The listing builds one solid part. Answer for the finished solid, in the listing's coordinates (mm). A direction names the side the tool comes from. Coordinates: 2 decimals unless noted, no trailing zeros. Loops run counter-clockwise (first coordinate to the right, second up) from the corner with the lowest first, then second, coordinate; pieces in that order, holes last. Notation, with made-up numbers: (43.5, 12) -> (81.5, 12) arc R10 ccw to (81.5, 30) -> close; hole circle Ø4 at (7.25, 39.25). An arc over 180 degrees is marked (long way). Answer in a Markdown table with one row per item.
```python
from build123d import *

# Parameters (mm, degrees)
AXIAL_PROFILE_MM_W     = 5
AXIAL_PROFILE_MM_H     = 34.4
AXIAL_HOLES_DEPTH      = 176.574514096
AXIAL_HOLES_DEPTH_BACK = 176.574514096
SKETCH2_R              = 1.65
CUT_EXTRUDE2_START     = 165.2
SKETCH3_R              = 1.65
CUT_EXTRUDE2_DEPTH     = 3.5


with BuildPart() as part:
    # Axial profile (mm) → Full revolution (revolve)
    with BuildSketch(Plane.XY, mode=Mode.PRIVATE) as full_revolution_sk:
        with Locations((166.2, 17.2)):
            Rectangle(AXIAL_PROFILE_MM_W, AXIAL_PROFILE_MM_H)
    revolve(full_revolution_sk.sketch.rotate(Axis((-110, 0, 0), (1, 0, 0)), 90), axis=Axis((-110, 0, 0), (1, 0, 0)))

    # Sketch2 → Axial holes (cut, two sides: drawn at the far end of the back side and taken through both)
    with BuildSketch(Plane(origin=(0, 0, 0), x_dir=(0, 0, -1), z_dir=(1, 0, 0)).offset(-AXIAL_HOLES_DEPTH_BACK)):
        with Locations((-29.4, 0)):
            Circle(SKETCH2_R)
        with Locations((14.7, -25.461146871)):
            Circle(SKETCH2_R)
        with Locations((14.7, 25.461146871)):
            Circle(SKETCH2_R)
    extrude(amount=AXIAL_HOLES_DEPTH + AXIAL_HOLES_DEPTH_BACK, mode=Mode.SUBTRACT)

    # Sketch3 → Cut-Extrude2 (cut)
    with BuildSketch(Plane(origin=(0, 0, 0), x_dir=(0, 0, -1), z_dir=(1, 0, 0)).offset(CUT_EXTRUDE2_START)):
        with Locations((29.4, 0)):
            Circle(SKETCH3_R)
        with Locations((-14.7, 25.461146871)):
            Circle(SKETCH3_R)
        with Locations((-14.7, -25.461146871)):
            Circle(SKETCH3_R)
    extrude(amount=CUT_EXTRUDE2_DEPTH, mode=Mode.SUBTRACT)


solid = part.part
```
Item 1: Determine the mould class of faces 1 (the face through (166.165, 0.496, 27.826)), 2 (the face through (168.7, 0, 0)), 3 (the face through (166.235, -1.513, -34.367)) for opening direction Z: +Z half, -Z half, draft (parallel to the pull), parting line (faces both ways), or undercut.
Findings below:
| item | result |
|---|---|
| face 1 | undercut |
| face 2 | draft |
| face 3 | parting line |
Item 2: Flat-ended cylindrical pins translate along their axes: pin 1 Ø1.5 at (x, y) = (167, 21) entering from +Z; pin 2 Ø3 at (y, z) = (25.46, 14.7) entering from +X; pin 3 Ø2.5 at (y, z) = (-25.46, -14.7) entering from -X; pin 4 Ø3 at (x, z) = (167.5, 18) entering from +Y. Find the tip coordinate at first contact, or state that the pin passes through.
Findings below:
| item | result |
|---|---|
| pin 1 | stops at z = 27.81 |
| pin 2 | stops at x = 165.2 |
| pin 3 | passes through |
| pin 4 | stops at y = 30.18 |
Item 3: A cutting plane is placed at D-D, the plane z = -29.4. Determine the outline of the cut face in (x, y), plus the area to 3 significant figures.
Findings below:
| item | result |
|---|---|
| outline | (163.7, -17.86) -> (168.7, -17.86) -> (168.7, -1.65) -> (165.2, -1.65) -> (165.2, 1.65) -> (168.7, 1.65) -> (168.7, 17.86) -> (163.7, 17.86) -> close |
| area | 167 mm2 |
Item 4: A tool of negligible diameter and unlimited length cuts with its end or side. For faces 4 (the face through (166.926, 26.576, 15.916)), 5 (the face through (163.7, 0, 0)), from which of +Z, -Z, +X, -X, +Y, -Y can it reach the whole face along a straight path? Write none if from no direction.
Findings below:
| item | result |
|---|---|
| face 4 | +X |
| face 5 | +Z, -Z, -X, +Y, -Y |
Item 5: Find the intervals of material crossed by probe 1 along Y at (x, z) = (166.3, 14.7); probe 2 along Y at (x, z) = (166.1, -13.5); probe 3 along Z at (x, y) = (167.45, 1), in increasing order.
Findings below:
| item | result |
|---|---|
| probe 1 | y = -31.1 to -27.11, -23.81 to 23.81, 27.11 to 31.1 |
| probe 2 | y = -31.64 to -26.59, -24.33 to 24.33, 26.59 to 31.64 |
| probe 3 | z = -34.39 to -30.71, -28.09 to 28.09, 30.71 to 34.39 |
Item 6: A cutting plane is placed at B-B, the plane z = -14.7. Determine the outline of the cut face in (x, y), plus the area to 3 significant figures.
Findings below:
| item | result |
|---|---|
| outline | (163.7, -31.1) -> (168.7, -31.1) -> (168.7, -27.11) -> (163.7, -27.11) -> close; (163.7, -23.81) -> (168.7, -23.81) -> (168.7, 23.81) -> (163.7, 23.81) -> close; (163.7, 27.11) -> (168.7, 27.11) -> (168.7, 31.1) -> (163.7, 31.1) -> close |
| area | 278 mm2 |
Item 7: A cutting plane is placed at A-A, the plane y = 0. Determine the outline of the cut face in (x, z), plus the area to 3 significant figures.
Findings below:
| item | result |
|---|---|
| outline | (163.7, -34.4) -> (168.7, -34.4) -> (168.7, -31.05) -> (165.2, -31.05) -> (165.2, -27.75) -> (168.7, -27.75) -> (168.7, 27.75) -> (163.7, 27.75) -> close; (163.7, 31.05) -> (168.7, 31.05) -> (168.7, 34.4) -> (163.7, 34.4) -> close |
| area | 316 mm2 |
Item 8: A cutting plane is placed at C-C, the plane x = 166.5. Determine the outline of the cut face in (y, z), plus the area to 3 significant figures.
Findings below:
| item | result |
|---|---|
| outline | circle Ø68.8 at (0, 0); hole circle Ø3.3 at (-25.46, -14.7); hole circle Ø3.3 at (-25.46, 14.7); hole circle Ø3.3 at (0, -29.4); hole circle Ø3.3 at (0, 29.4); hole circle Ø3.3 at (25.46, -14.7); hole circle Ø3.3 at (25.46, 14.7) |
| area | 3,670 mm2 |
